from build123d import *

# Parameters (mm, degrees)
SKETCH_5_OUTSIDE_W  = 11.028
SKETCH_5_OUTSIDE_H  = 11.028
CUT_EXTRUDE_6_DEPTH = 1.1
CHAMFER_4_SIZE      = 0.3


with BuildPart() as part:
    # Эскиз3 → Повернуть1 (revolve)
    with BuildSketch(Plane.XY):
        Polygon((1.1, 2), (1.1, 3.15), (1.006217783, 3.5), (-1.006217783, 3.5), (-1.1, 3.15), (-1.1, 2), align=None)
    revolve(axis=Axis((-2.78527838, 0, 0), (1, 0, 0)))

    # Эскиз5 outside → Вырез-Вытянуть6 (cut, symmetric)
    with BuildSketch(Plane(origin=(0, 0, 0), x_dir=(0, 0, -1), z_dir=(1, 0, 0))):
        Rectangle(SKETCH_5_OUTSIDE_W, SKETCH_5_OUTSIDE_H)
        Polygon((0, 3.5), (-3.031088913, 1.75), (-3.031088913, -1.75), (0, -3.5), (3.031088913, -1.75), (3.031088913, 1.75), align=None, mode=Mode.SUBTRACT)
    extrude(amount=CUT_EXTRUDE_6_DEPTH, both=True, mode=Mode.SUBTRACT)

    # Фаска4
    chamfer_4_edges = [part.edges().sort_by_distance(p)[0] for p in [
        (-1.1, -2, 0),
        (1.1, -2, 0),
    ]]
    chamfer(chamfer_4_edges, length=CHAMFER_4_SIZE)


solid = part.part
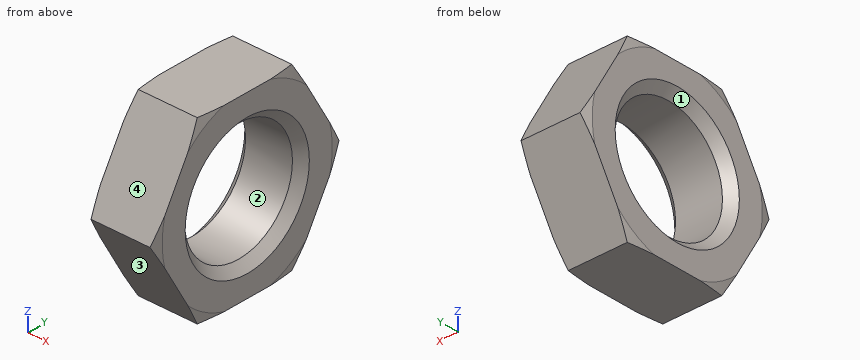
Build history of the part. All positions in model axes, mm. Face numbers are marked on the shaded views. Give positions to 0.01 mm unless a question says otherwise; leave off trailing zeros. Order: outer loops, then holes, each group sorted by start corner. A loop starts at its lowest first (then second) coordinate and runs counter-clockwise, first axis right, second up. Notation, with made-up numbers: M 25.5,46.25 L 36.5,46.25 A18 cw 36.5,70.25 Z; hole C 34.5,85.25 d2. An arc over 180 degrees is marked long. Put each result on its own line as item: value.
Item 1: Flat gauge pins, fed straight in: pin 1 Ø1 at (y, z) = (-0.5, -1.5) entering from +X; pin 2 Ø1 at (y, z) = (-1, -0.5) entering from +X. Where does each tip first touch, or does it go through?
From the geometry:
pin 1: stops at x = 0.88
pin 2: passes through
Item 2: Slice it at A-A, the plane y = 0. Write the cut outline in (x, z).
From the geometry:
outline: M -1.1,-3.03 L 1.1,-3.03 L 1.1,-2.3 L 0.8,-2 L -0.8,-2 L -1.1,-2.3 Z; M -1.1,2.3 L -0.8,2 L 0.8,2 L 1.1,2.3 L 1.1,3.03 L -1.1,3.03 Z
Item 3: Slice it at B-B, the plane x = 0.3. Write the cut outline in (y, z), plus the area to 3 significant figures.
From the geometry:
outline: M -3.5,0 L -1.75,-3.03 L 1.75,-3.03 L 3.5,0 L 1.75,3.03 L -1.75,3.03 Z; hole C 0,0 d4
area: 19.3 mm2
Item 4: Two-plate mould, pull along Z, no slides. Class the marked faces 1, 2, 3 and 4: +Z half, -Z half, draft (parallel to the pull), parting line (faces both ways), or undercut.
From the geometry:
face 1: undercut
face 2: undercut
face 3: -Z half
face 4: +Z half
Item 5: Probe line 1 (Z direction, x = 0.5, y = 0); line 2 (Y direction, x = 0.7, z = 0.25); line 3 (Y direction, x = 0.1, z = 1). List the from-to ranges inside material, lowest first. Write a range as [from, to].
From the geometry:
line 1: z = [-3.03, -2], [2, 3.03]
line 2: y = [-3.36, -1.98], [1.98, 3.36]
line 3: y = [-2.92, -1.73], [1.73, 2.92]
